Input: part model. Units: mm. Frame: model coordinates. Face numbers are marked on the shaded views. A direction names the side the tool comes from. Give positions to 0.01 mm unless a question says otherwise; leave off trailing zeros. Loops run counter-clockwise (first coordinate to the right, second up) from the corner with the lowest first, then second, coordinate; pieces in that order, holes last. Notation, with made-up numbers: (67.5, 81) - (121.5, 81) arc R23 ccw to (121.5, 91) - close; hole circle Ø8 at (-34, 18.25). An arc over 180 degrees is marked (long way). Answer as a JSON object with one key per item and string values. Group by question number.
(1) Section query C-C (z = -8). Return loops of the section in (x, y).
(2) Section query B-B (y = 26.5). Return loops of the section in (x, z), plus the area to 3 significant figures.
(3) Section query A-A (x = 0). Return loops of the section in (y, z), plus the area to 3 significant figures.
(4) Mould query, pull axis X, two halves, no side actions, for the marked faces 3, 4, 5 and 6. Classes: +X half, -X half, draft (parallel to the pull), parting line (faces both ways), or undercut.
(5) Access query for the marked faces 1 and 2. Directions: +Z, -Z, +X, -X, +Y, -Y. A direction counts if a zero-diameter tool reaches every point of the face in a straight line with its end or side. Return the directions, or none.
(6) Section query D-D (x = 4). Return loops of the section in (y, z).
(7) Material intervals for L1, parallel to Y at x = 0, z = -17; L2, parallel to X at y = -11, z = 8.5; L3, parallel to Z at x = 0, y = -14, sorted ascending.
(8) Pin query (flat end, axial travel): P1, Ø6, axis at x = 6, z = -17.5, coming from the -Y side; P2, Ø8, axis at x = 4, z = -1.5, coming from the -Y side; P3, Ø1.5, axis at y = 8, z = -25.5, coming from the -X side; P4, Ø5, axis at x = 3, y = 14.5, coming from the -Z side. Return the tip coordinate at first contact, or that it passes through.
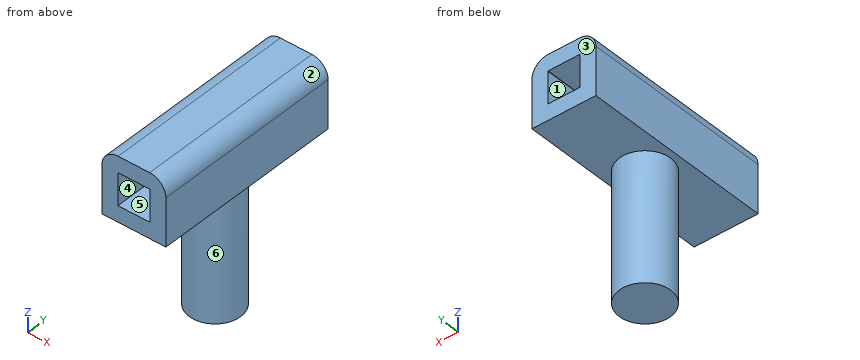
```python
from build123d import *

# Parameters (mm, degrees)
F0_R     = 8
F1_DEPTH = 40
F2_W     = 20
F2_H     = 60
F3_DEPTH = 20
F4_R     = 5.08
F6_T     = -5


with BuildPart() as f1:
    # F0 (on Top) → F1 (new body)
    with BuildSketch(Plane.XY):
        Circle(F0_R)
    extrude(amount=-F1_DEPTH)

    # F2 (on Top) + F0 (on Top) → F3 (join)
    with BuildSketch(Plane.XY):
        Rectangle(F2_W, F2_H)
    with BuildSketch(Plane.XY):
        Circle(F0_R)
    extrude(amount=F3_DEPTH)

    # F4
    f4_edges = [f1.edges().sort_by_distance(p)[0] for p in [
        (-10, 0, 20),
        (10, 0, 20),
    ]]
    fillet(f4_edges, radius=F4_R)

    # F6
    f6_openings = [f1.faces().sort_by_distance(p)[0] for p in [
        (0, -30, 9.747524),
        (0, 30, 9.747524),
    ]]
    offset(amount=F6_T, openings=f6_openings, kind=Kind.INTERSECTION)


solid = f1.part
```
Recorded:
{
 "1": {"outline": "circle Ø16 at (0, 0); hole circle Ø6 at (0, 0)"},
 "2": {"outline": "(-10, 0) - (10, 0) - (10, 14.92) arc R5.08 ccw to (4.92, 20) - (-4.92, 20) arc R5.08 ccw to (-10, 14.92) - close; hole (-5, 5) - (5, 5) - (5, 14.92) arc R0.08 ccw to (4.92, 15) - (-4.92, 15) arc R0.08 ccw to (-5, 14.92) - close", "area": "289 mm^2"},
 "3": {"outline": "(-30, 0) - (-8, 0) - (-8, -40) - (8, -40) - (8, 0) - (30, 0) - (30, 5) - (3, 5) - (3, -35) - (-3, -35) - (-3, 5) - (-30, 5) - close; (-30, 15) - (30, 15) - (30, 20) - (-30, 20) - close", "area": "1,000 mm^2"},
 "4": {"face 3": "draft", "face 4": "undercut", "face 5": "undercut", "face 6": "parting line"},
 "5": {"face 1": "+Y, -Y", "face 2": "+Z, +X, +Y, -Y"},
 "6": {"outline": "(-30, 0) - (-6.93, 0) - (-6.93, -40) - (6.93, -40) - (6.93, 0) - (30, 0) - (30, 5) - (-30, 5) - close; (-30, 15) - (30, 15) - (30, 20) - (-30, 20) - close"},
 "7": {"L1": "y = -8 to -3, 3 to 8", "L2": "x = -10 to -5, 5 to 10", "L3": "z = 0 to 5, 15 to 20"},
 "8": {"P1": "stops at y = -7.42", "P2": "stops at y = -30", "P3": "stops at x = -3.38", "P4": "stops at z = 0"}
}
